Here's how the part is built. I have some questions about the finished solid (model axes, mm). A direction names the side the tool comes from. Give positions to 0.01 mm unless a question says otherwise; leave off trailing zeros. Order: outer loops, then holes, each group sorted by start corner. A loop starts at its lowest first (then second) coordinate and runs counter-clockwise, first axis right, second up.
from build123d import *

# Parameters (mm, degrees)
F1_DEPTH = 12.7


with BuildPart() as f1:
    # F0 (on Top) → F1 (new body, symmetric)
    with BuildSketch(Plane.XY):
        with BuildLine():
            ThreePointArc((75.134213, -12.7), (75.933086, -6.372321), (76.2, 0))
            ThreePointArc((76.2, 0), (75.933086, 6.372321), (75.134213, 12.7))
            ThreePointArc((75.134213, 12.7), (53.881537, 53.881537), (12.7, 75.134213))
            ThreePointArc((12.7, 75.134213), (0, 76.2), (-12.7, 75.134213))
            ThreePointArc((-12.7, 75.134213), (-53.881537, 53.881537), (-75.134213, 12.7))
            ThreePointArc((-75.134213, 12.7), (-76.2, 0), (-75.134213, -12.7))
            ThreePointArc((-75.134213, -12.7), (-53.881537, -53.881537), (-12.7, -75.134213))
            ThreePointArc((-12.7, -75.134213), (0, -76.2), (12.7, -75.134213))
            ThreePointArc((12.7, -75.134213), (53.881537, -53.881537), (75.134213, -12.7))
        make_face()
        Polygon((-25.670162, -70.528192), (-26.787991, -64.18867), (-20.73889, -66.390362), align=None, mode=Mode.SUBTRACT)
        Polygon((-64.999133, -37.527267), (-61.780473, -31.952385), (-58.561814, -37.527267), align=None, mode=Mode.SUBTRACT)
        with BuildLine():
            Line((-34.771706, -12.7), (-19.05, -12.7))
            ThreePointArc((-19.05, -12.7), (-14.559872, -14.559872), (-12.7, -19.05))
            Line((-12.7, -19.05), (-12.7, -34.771706))
            Line((-12.7, -34.771706), (-12.7, -45.838683))
            Line((-12.7, -45.838683), (-12.7, -53.881537))
            ThreePointArc((-12.7, -53.881537), (-15.383826, -59.06629), (-21.166667, -59.868374))
            ThreePointArc((-21.166667, -59.868374), (-44.901281, -44.901281), (-59.868374, -21.166667))
            ThreePointArc((-59.868374, -21.166667), (-59.06629, -15.383826), (-53.881537, -12.7))
            Line((-53.881537, -12.7), (-45.838683, -12.7))
            Line((-45.838683, -12.7), (-34.771706, -12.7))
        make_face(mode=Mode.SUBTRACT)
        Polygon((25.670162, -70.528192), (20.73889, -66.390362), (26.787991, -64.18867), align=None, mode=Mode.SUBTRACT)
        with BuildLine():
            ThreePointArc((12.7, -19.05), (14.559872, -14.559872), (19.05, -12.7))
            Line((19.05, -12.7), (34.771706, -12.7))
            Line((34.771706, -12.7), (45.838683, -12.7))
            Line((45.838683, -12.7), (53.881537, -12.7))
            ThreePointArc((53.881537, -12.7), (59.06629, -15.383826), (59.868374, -21.166667))
            ThreePointArc((59.868374, -21.166667), (44.901281, -44.901281), (21.166667, -59.868374))
            ThreePointArc((21.166667, -59.868374), (15.383826, -59.06629), (12.7, -53.881537))
            Line((12.7, -53.881537), (12.7, -45.838683))
            Line((12.7, -45.838683), (12.7, -34.771706))
            Line((12.7, -34.771706), (12.7, -19.05))
        make_face(mode=Mode.SUBTRACT)
        Polygon((64.999133, -37.527267), (58.561814, -37.527267), (61.780473, -31.952385), align=None, mode=Mode.SUBTRACT)
        Polygon((-73.914287, 13.033083), (-67.865185, 15.234776), (-68.983014, 8.895254), align=None, mode=Mode.SUBTRACT)
        with BuildLine():
            ThreePointArc((-59.868374, 21.166667), (-44.901281, 44.901281), (-21.166667, 59.868374))
            ThreePointArc((-21.166667, 59.868374), (-15.383826, 59.06629), (-12.7, 53.881537))
            Line((-12.7, 53.881537), (-12.7, 45.838683))
            Line((-12.7, 45.838683), (-12.7, 34.771706))
            Line((-12.7, 34.771706), (-12.7, 19.05))
            ThreePointArc((-12.7, 19.05), (-14.559872, 14.559872), (-19.05, 12.7))
            Line((-19.05, 12.7), (-34.771706, 12.7))
            Line((-34.771706, 12.7), (-45.838683, 12.7))
            Line((-45.838683, 12.7), (-53.881537, 12.7))
            ThreePointArc((-53.881537, 12.7), (-59.06629, 15.383826), (-59.868374, 21.166667))
        make_face(mode=Mode.SUBTRACT)
        Polygon((-48.244124, 57.495109), (-42.195023, 55.293416), (-47.126296, 51.155587), align=None, mode=Mode.SUBTRACT)
        with BuildLine():
            ThreePointArc((0, 12.7), (8.980256, 8.980256), (12.7, 0))
            ThreePointArc((12.7, 0), (8.980256, -8.980256), (0, -12.7))
            ThreePointArc((0, -12.7), (-8.980256, -8.980256), (-12.7, 0))
            ThreePointArc((-12.7, 0), (-8.980256, 8.980256), (0, 12.7))
        make_face(mode=Mode.SUBTRACT)
        with BuildLine():
            ThreePointArc((19.05, 12.7), (14.559872, 14.559872), (12.7, 19.05))
            Line((12.7, 19.05), (12.7, 34.771706))
            Line((12.7, 34.771706), (12.7, 45.838683))
            Line((12.7, 45.838683), (12.7, 53.881537))
            ThreePointArc((12.7, 53.881537), (15.383826, 59.06629), (21.166667, 59.868374))
            ThreePointArc((21.166667, 59.868374), (44.901281, 44.901281), (59.868374, 21.166667))
            ThreePointArc((59.868374, 21.166667), (59.06629, 15.383826), (53.881537, 12.7))
            Line((53.881537, 12.7), (45.838683, 12.7))
            Line((45.838683, 12.7), (34.771706, 12.7))
            Line((34.771706, 12.7), (19.05, 12.7))
        make_face(mode=Mode.SUBTRACT)
        Polygon((73.914287, 13.033083), (68.983014, 8.895254), (67.865185, 15.234776), align=None, mode=Mode.SUBTRACT)
        Polygon((0, 75.054534), (3.21866, 69.479652), (-3.21866, 69.479652), align=None, mode=Mode.SUBTRACT)
        Polygon((48.244124, 57.495109), (47.126296, 51.155587), (42.195023, 55.293416), align=None, mode=Mode.SUBTRACT)
    extrude(amount=F1_DEPTH, both=True)


solid = f1.part
Q1. If we section it at B-B on x = -17: List the corners of the cut face in (y, z) for me.
Filled sheet:
outline: (-74.28, -12.7) - (-59.89, -12.7) - (-59.89, 12.7) - (-74.28, 12.7) - close; (-13.04, -12.7) - (13.04, -12.7) - (13.04, 12.7) - (-13.04, 12.7) - close; (59.89, -12.7) - (74.28, -12.7) - (74.28, 12.7) - (59.89, 12.7) - close
Q2. If we section it at C-C on y = 44: List the corners of the cut face in (x, z) for me, plus the area to 3 significant figures.
Filled sheet:
outline: (-62.21, -12.7) - (-45.78, -12.7) - (-45.78, 12.7) - (-62.21, 12.7) - close; (-12.7, -12.7) - (12.7, -12.7) - (12.7, 12.7) - (-12.7, 12.7) - close; (45.78, -12.7) - (62.21, -12.7) - (62.21, 12.7) - (45.78, 12.7) - close
area: 1,480 mm2
Q3. If we section it at D-D on z = -10.5: Give the number of separate pieces and of enclosed holes in the cut face, plus the area to 3 significant figures.
Filled sheet:
separate pieces: 1
enclosed holes: 14
area: 10,800 mm2
Q4. I need wall thicknesses on L1, parallel to X at y = -42, z = -1.5; L2, parallel to Y at x = -41.5, z = -7; L3, parallel to Y at x = -53, z = -10.25 (3 decimals). Which ranges of each line are inside material? Lowest first, please.
Filled sheet:
L1: x = -63.58 to -47.63, -12.7 to 12.7, 47.63 to 63.58
L2: y = -63.91 to -48.06, -12.7 to 12.7, 48.06 to 63.91
L3: y = -54.749 to -34.975, -12.7 to 12.7, 34.975 to 54.749
Q5. If we section it at A-A on y = 6: List the corners of the cut face in (x, z) for me, plus the area to 3 significant figures.
Filled sheet:
outline: (-75.96, -12.7) - (-11.19, -12.7) - (-11.19, 12.7) - (-75.96, 12.7) - close; (11.19, -12.7) - (75.96, -12.7) - (75.96, 12.7) - (11.19, 12.7) - close
area: 3,290 mm2
Q6. For faces 4 (the face through (-54.35, -53.41, 0.18)), 5 (the face through (-15.453, 59.115, 0.178)), which set-ups out of +Z, -Z, +X, -X, +Y, -Y let a thin tool reach every point of the face, with its end or its side?
Filled sheet:
face 4: +Z, -Z, -X, -Y
face 5: +Z, -Z
Q7. Thinking about a two-plate mould opening in X: for faces 1 (the face through (44.6, 45.2, 0.2)), 2 (the face through (-1, -16, -12.7)), 3 (the face through (-76.2, 0.2, 0.2)), which applies, released by +X, released by -X, zero draft, split by the parting line, or undercut?
Filled sheet:
face 1: undercut
face 2: zero draft
face 3: released by -X
Q8. I'm going to push flat-ended pins straight in: P1, Ø12.5, axis at x = -40.5, z = -5, coming from the -Y side; P2, Ø12.5, axis at x = -44.5, z = -3.5, coming from the +Y side; P3, Ø2, axis at x = -8, z = -6.5, coming from the +Y side; P4, Ø8, axis at x = -41.5, y = 45, coming from the -Z side. Where does each tip first touch, or does it pass through?
Filled sheet:
P1: stops at y = -68.07
P2: stops at y = 65.9
P3: stops at y = 75.88
P4: stops at z = -12.7
